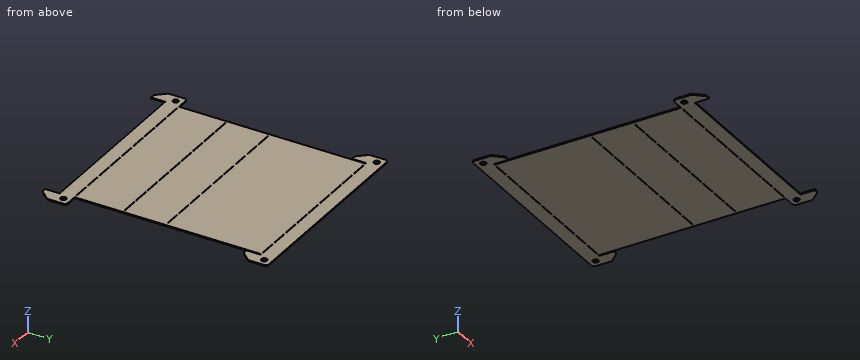
from build123d import *

# Parameters (mm, degrees)
F0_R     = 5
F1_DEPTH = 2


with BuildPart() as f1:
    # F0 (on Top) → F1 (new body)
    with BuildSketch(Plane.XY):
        with BuildLine():
            Line((-156.5, 353), (-154.5, 353))
            Line((-154.5, 353), (-154.5, 378))
            Line((-154.5, 378), (-174.5, 378))
            ThreePointArc((-174.5, 378), (-178.0355339059, 376.5355339059), (-179.5, 373))
            Line((-179.5, 373), (-179.5, 353))
            Line((-179.5, 353), (-156.5, 353))
        make_face()
        with Locations((-166.5, 365.5)):
            Circle(F0_R, mode=Mode.SUBTRACT)
        with BuildLine():
            Line((-156.5, 328), (-156.5, 353))
            Line((-156.5, 353), (-179.5, 353))
            Line((-179.5, 353), (-179.5, 346.8905226992))
            ThreePointArc((-179.5, 346.8905226992), (-179.1768550536, 345.1221825713), (-178.2491892768, 343.5824145137))
            Line((-178.2491892768, 343.5824145137), (-165.9928457187, 329.6918918146))
            ThreePointArc((-165.9928457187, 329.6918918146), (-164.300287069, 328.4425587811), (-162.2436564419, 328))
            Line((-162.2436564419, 328), (-156.5, 328))
        make_face()
        Polygon((-154.5, 378), (-154.5, 353), (-148.5, 353), (-148.5, 353.5), (-120.8, 353.5), (-120.8, 353), (-114.8, 353), (-114.8, 353.5), (-87.1, 353.5), (-87.1, 353), (-81.1, 353), (-81.1, 353.5), (-53.4, 353.5), (-53.4, 353), (-47.4, 353), (-47.4, 353.5), (-19.7, 353.5), (-19.7, 353), (-13.7, 353), (-13.7, 353.5), (0, 353.5), (0, 378), align=None)
        Polygon((-154.5, 353), (-154.5, 110), (-148.5, 110), (-148.5, 110.5), (-120.8, 110.5), (-120.8, 110), (-114.8, 110), (-114.8, 110.5), (-87.1, 110.5), (-87.1, 110), (-81.1, 110), (-81.1, 110.5), (-53.4, 110.5), (-53.4, 110), (-47.4, 110), (-47.4, 110.5), (-19.7, 110.5), (-19.7, 110), (-13.7, 110), (-13.7, 110.5), (0, 110.5), (0, 184.5), (-13.7, 184.5), (-13.7, 185), (-13.7, 185.5), (0, 185.5), (0, 352.5), (-13.7, 352.5), (-13.7, 353), (-19.7, 353), (-19.7, 352.5), (-47.4, 352.5), (-47.4, 353), (-53.4, 353), (-53.4, 352.5), (-81.1, 352.5), (-81.1, 353), (-87.1, 353), (-87.1, 352.5), (-114.8, 352.5), (-114.8, 353), (-120.8, 353), (-120.8, 352.5), (-148.5, 352.5), (-148.5, 353), align=None)
        Polygon((-120.8, 185.5), (-120.8, 185), (-120.8, 184.5), (-148.5, 184.5), (-148.5, 185), (-148.5, 185.5), align=None, mode=Mode.SUBTRACT)
        Polygon((-87.1, 185.5), (-87.1, 185), (-87.1, 184.5), (-114.8, 184.5), (-114.8, 185), (-114.8, 185.5), align=None, mode=Mode.SUBTRACT)
        Polygon((-53.4, 185.5), (-53.4, 185), (-53.4, 184.5), (-81.1, 184.5), (-81.1, 185), (-81.1, 185.5), align=None, mode=Mode.SUBTRACT)
        Polygon((-19.7, 185.5), (-19.7, 185), (-19.7, 184.5), (-47.4, 184.5), (-47.4, 185), (-47.4, 185.5), align=None, mode=Mode.SUBTRACT)
        Polygon((148.5, 353), (154.5, 353), (154.5, 378), (0, 378), (0, 353.5), (13.7, 353.5), (13.7, 353), (19.7, 353), (19.7, 353.5), (47.4, 353.5), (47.4, 353), (53.4, 353), (53.4, 353.5), (81.1, 353.5), (81.1, 353), (87.1, 353), (87.1, 353.5), (114.8, 353.5), (114.8, 353), (120.8, 353), (120.8, 353.5), (148.5, 353.5), align=None)
        Polygon((148.5, 110), (154.5, 110), (154.5, 353), (148.5, 353), (148.5, 352.5), (120.8, 352.5), (120.8, 353), (114.8, 353), (114.8, 352.5), (87.1, 352.5), (87.1, 353), (81.1, 353), (81.1, 352.5), (53.4, 352.5), (53.4, 353), (47.4, 353), (47.4, 352.5), (19.7, 352.5), (19.7, 353), (13.7, 353), (13.7, 352.5), (0, 352.5), (0, 185.5), (13.7, 185.5), (13.7, 185), (13.7, 184.5), (0, 184.5), (0, 110.5), (13.7, 110.5), (13.7, 110), (19.7, 110), (19.7, 110.5), (47.4, 110.5), (47.4, 110), (53.4, 110), (53.4, 110.5), (81.1, 110.5), (81.1, 110), (87.1, 110), (87.1, 110.5), (114.8, 110.5), (114.8, 110), (120.8, 110), (120.8, 110.5), (148.5, 110.5), align=None)
        Polygon((19.7, 184.5), (19.7, 185), (19.7, 185.5), (47.4, 185.5), (47.4, 185), (47.4, 184.5), align=None, mode=Mode.SUBTRACT)
        Polygon((53.4, 184.5), (53.4, 185), (53.4, 185.5), (81.1, 185.5), (81.1, 185), (81.1, 184.5), align=None, mode=Mode.SUBTRACT)
        Polygon((87.1, 184.5), (87.1, 185), (87.1, 185.5), (114.8, 185.5), (114.8, 185), (114.8, 184.5), align=None, mode=Mode.SUBTRACT)
        Polygon((120.8, 184.5), (120.8, 185), (120.8, 185.5), (148.5, 185.5), (148.5, 185), (148.5, 184.5), align=None, mode=Mode.SUBTRACT)
        with BuildLine():
            Line((154.5, 378), (154.5, 353))
            Line((154.5, 353), (156.5, 353))
            Line((156.5, 353), (179.5, 353))
            Line((179.5, 353), (179.5, 373))
            ThreePointArc((179.5, 373), (178.0355339059, 376.5355339059), (174.5, 378))
            Line((174.5, 378), (154.5, 378))
        make_face()
        with Locations((166.5, 365.5)):
            Circle(F0_R, mode=Mode.SUBTRACT)
        with BuildLine():
            Line((179.5, 353), (156.5, 353))
            Line((156.5, 353), (156.5, 328))
            Line((156.5, 328), (162.2436564419, 328))
            ThreePointArc((162.2436564419, 328), (164.300287069, 328.4425587811), (165.9928457187, 329.6918918146))
            Line((165.9928457187, 329.6918918146), (178.2491892768, 343.5824145137))
            ThreePointArc((178.2491892768, 343.5824145137), (179.1768550536, 345.1221825713), (179.5, 346.8905226992))
            Line((179.5, 346.8905226992), (179.5, 353))
        make_face()
        with BuildLine():
            Line((-156.5, -25), (-156.5, 0))
            Line((-156.5, 0), (-179.5, 0))
            Line((-179.5, 0), (-179.5, -6.1094773008))
            ThreePointArc((-179.5, -6.1094773008), (-179.1768550536, -7.8778174287), (-178.2491892768, -9.4175854863))
            Line((-178.2491892768, -9.4175854863), (-165.9928457187, -23.3081081854))
            ThreePointArc((-165.9928457187, -23.3081081854), (-164.300287069, -24.5574412189), (-162.2436564419, -25))
            Line((-162.2436564419, -25), (-156.5, -25))
        make_face()
        with BuildLine():
            Line((-156.5, 0), (-154.5, 0))
            Line((-154.5, 0), (-154.5, 25))
            Line((-154.5, 25), (-174.5, 25))
            ThreePointArc((-174.5, 25), (-178.0355339059, 23.5355339059), (-179.5, 20))
            Line((-179.5, 20), (-179.5, 0))
            Line((-179.5, 0), (-156.5, 0))
        make_face()
        with Locations((-166.5, 12.5)):
            Circle(F0_R, mode=Mode.SUBTRACT)
        Polygon((-154.5, 0), (0, 0), (0, 24.5), (-13.7, 24.5), (-13.7, 25), (-19.7, 25), (-19.7, 24.5), (-47.4, 24.5), (-47.4, 25), (-53.4, 25), (-53.4, 24.5), (-81.1, 24.5), (-81.1, 25), (-87.1, 25), (-87.1, 24.5), (-114.8, 24.5), (-114.8, 25), (-120.8, 25), (-120.8, 24.5), (-148.5, 24.5), (-148.5, 25), (-154.5, 25), align=None)
        Polygon((-154.5, 110), (-154.5, 25), (-148.5, 25), (-148.5, 25.5), (-120.8, 25.5), (-120.8, 25), (-114.8, 25), (-114.8, 25.5), (-87.1, 25.5), (-87.1, 25), (-81.1, 25), (-81.1, 25.5), (-53.4, 25.5), (-53.4, 25), (-47.4, 25), (-47.4, 25.5), (-19.7, 25.5), (-19.7, 25), (-13.7, 25), (-13.7, 25.5), (0, 25.5), (0, 109.5), (-13.7, 109.5), (-13.7, 110), (-19.7, 110), (-19.7, 109.5), (-47.4, 109.5), (-47.4, 110), (-53.4, 110), (-53.4, 109.5), (-81.1, 109.5), (-81.1, 110), (-87.1, 110), (-87.1, 109.5), (-114.8, 109.5), (-114.8, 110), (-120.8, 110), (-120.8, 109.5), (-148.5, 109.5), (-148.5, 110), align=None)
        Polygon((148.5, 25), (154.5, 25), (154.5, 110), (148.5, 110), (148.5, 109.5), (120.8, 109.5), (120.8, 110), (114.8, 110), (114.8, 109.5), (87.1, 109.5), (87.1, 110), (81.1, 110), (81.1, 109.5), (53.4, 109.5), (53.4, 110), (47.4, 110), (47.4, 109.5), (19.7, 109.5), (19.7, 110), (13.7, 110), (13.7, 109.5), (0, 109.5), (0, 25.5), (13.7, 25.5), (13.7, 25), (19.7, 25), (19.7, 25.5), (47.4, 25.5), (47.4, 25), (53.4, 25), (53.4, 25.5), (81.1, 25.5), (81.1, 25), (87.1, 25), (87.1, 25.5), (114.8, 25.5), (114.8, 25), (120.8, 25), (120.8, 25.5), (148.5, 25.5), align=None)
        Polygon((0, 24.5), (0, 0), (154.5, 0), (154.5, 25), (148.5, 25), (148.5, 24.5), (120.8, 24.5), (120.8, 25), (114.8, 25), (114.8, 24.5), (87.1, 24.5), (87.1, 25), (81.1, 25), (81.1, 24.5), (53.4, 24.5), (53.4, 25), (47.4, 25), (47.4, 24.5), (19.7, 24.5), (19.7, 25), (13.7, 25), (13.7, 24.5), align=None)
        with BuildLine():
            Line((154.5, 25), (154.5, 0))
            Line((154.5, 0), (156.5, 0))
            Line((156.5, 0), (179.5, 0))
            Line((179.5, 0), (179.5, 20))
            ThreePointArc((179.5, 20), (178.0355339059, 23.5355339059), (174.5, 25))
            Line((174.5, 25), (154.5, 25))
        make_face()
        with Locations((166.5, 12.5)):
            Circle(F0_R, mode=Mode.SUBTRACT)
        with BuildLine():
            Line((179.5, 0), (156.5, 0))
            Line((156.5, 0), (156.5, -25))
            Line((156.5, -25), (162.2436564419, -25))
            ThreePointArc((162.2436564419, -25), (164.300287069, -24.5574412189), (165.9928457187, -23.3081081854))
            Line((165.9928457187, -23.3081081854), (178.2491892768, -9.4175854863))
            ThreePointArc((178.2491892768, -9.4175854863), (179.1768550536, -7.8778174287), (179.5, -6.1094773008))
            Line((179.5, -6.1094773008), (179.5, 0))
        make_face()
    extrude(amount=F1_DEPTH)


solid = f1.part
Source: CAD feature listing. Evaluate the final solid. Frame: model axes, mm. Coordinates: 2 decimals unless noted, no trailing zeros. Write each loop counter-clockwise with the first axis right and the second up, starting at its lowest first coordinate (ties: lowest second). Pieces come first, ordered by that corner, then holes. Notation, with made-up numbers: M -7.75,68.25 L 38.25,68.25 A19 ccw 38.25,100.25 Z; hole C -15,24 d9. An arc over 180 degrees is marked long. Use a Markdown table: item, result.
1) Section A-A, the plane y = 12.5. Output: boundary loops of the cut face in (x, z), then the cut area to 3 significant figures.
Conclusion:
| item | result |
|---|---|
| outline | M -179.5,0 L -171.5,0 L -171.5,2 L -179.5,2 Z; M -161.5,0 L 161.5,0 L 161.5,2 L -161.5,2 Z; M 171.5,0 L 179.5,0 L 179.5,2 L 171.5,2 Z |
| area | 678 mm^2 |
2) Ray query, L1, parallel to Y at x = 54, z = 1.1; L2, parallel to X at y = 365.5, z = 1.65; L3, parallel to Y at x = 166.5, z = 1.5. Return the intervals inside material, ascending.
Conclusion:
| item | result |
|---|---|
| L1 | y = 0 to 24.5, 25.5 to 109.5, 110.5 to 184.5, 185.5 to 352.5, 353.5 to 378 |
| L2 | x = -179.5 to -171.5, -161.5 to 161.5, 171.5 to 179.5 |
| L3 | y = -22.73 to 7.5, 17.5 to 25, 330.27 to 360.5, 370.5 to 378 |
3) Section B-B, the plane z = 0.85. Give the number of separate pieces and of enclosed holes in the cut face, then the cut area to 3 significant figures.
Conclusion:
| item | result |
|---|---|
| separate pieces | 1 |
| enclosed holes | 40 |
| area | 120,000 mm^2 |
4) First-contact query: pin 1 Ø4 at (x, y) = (62.5, 174.5) entering from -Z; pin 2 Ø1 at (y, z) = (230, 1) entering from -X; pin 3 Ø0.5 at (y, z) = (110, 1) entering from +X; pin 4 Ø1 at (x, z) = (-28.5, 1) entering from -Y. Flat tips, straight axial feed; report the tip coordinate or a pass-through.
Conclusion:
| item | result |
|---|---|
| pin 1 | stops at z = 0 |
| pin 2 | stops at x = -154.5 |
| pin 3 | stops at x = 154.5 |
| pin 4 | stops at y = 0 |
5) Section C-C, the plane y = 256.5. Output: boundary loops of the cut face in (x, z).
Conclusion:
| item | result |
|---|---|
| outline | M -154.5,0 L 154.5,0 L 154.5,2 L -154.5,2 Z |
